Check sheet for the modelled part. Datum: model origin and axes. Units: mm. A direction names the side the tool comes from. Round coordinates to 2 decimals unless told otherwise and drop trailing zeros. Answer in a Markdown table with one row per item.
```python
from build123d import *

# Parameters (mm, degrees)
SKETCH_1_R          = 0.7
EXTRUDE_1_DEPTH     = 11
SKETCH_3_W          = 21.5
SKETCH_3_H          = 10
EXTRUDE_2_DEPTH     = 1.6
SKETCH_4_W          = 5
SKETCH_4_H          = 5
CUT_EXTRUDE_1_DEPTH = 1
CUT_EXTRUDE_2_REACH = 62.995
SKETCH_5_R          = 1.5
SKETCH_5_W          = 8
SKETCH_5_H          = 3
SKETCH_6_W          = 9.004768993
SKETCH_6_H          = 22
SKETCH_6_H_2        = 21.052305639
CUT_EXTRUDE_3_DEPTH = 1
SKETCH_7_W          = 5.5
SKETCH_7_H          = 20
SKETCH_7_W_2        = 4.9
SKETCH_7_W_3        = 2
SKETCH_7_H_2        = 2
EXTRUDE_4_DEPTH     = 2
FILLET_2_R          = 0.5
CUT_EXTRUDE_4_REACH = 62.994
SKETCH_9_R          = 5.5
FILLET_3_R          = 3


with BuildPart() as part:
    # Эскиз1 → Бобышка-Вытянуть1 (new body)
    with BuildSketch(Plane.XY):
        with BuildLine():
            Line((-15.979444254, 30.494289473), (15.979444254, 30.494289473))
            ThreePointArc((15.979444254, 30.494289473), (17.393657817, 29.908503035), (17.979444254, 28.494289473))
            Line((17.979444254, 28.494289473), (17.979444254, -28.500000343))
            ThreePointArc((17.979444254, -28.500000343), (17.393657817, -29.914213905), (15.979444254, -30.500000343))
            Line((15.979444254, -30.500000343), (-15.979444254, -30.500000343))
            ThreePointArc((-15.979444254, -30.500000343), (-17.393657817, -29.914213905), (-17.979444254, -28.500000343))
            Line((-17.979444254, -28.500000343), (-17.979444254, 28.494289473))
            ThreePointArc((-17.979444254, 28.494289473), (-17.393657817, 29.908503035), (-15.979444254, 30.494289473))
        make_face()
        with Locations((-15.979444254, 28.500000343)):
            Circle(SKETCH_1_R, mode=Mode.SUBTRACT)
        with Locations((16.01925313, 28.489204167)):
            Circle(SKETCH_1_R, mode=Mode.SUBTRACT)
        with Locations((16.028296267, -28.484120661)):
            Circle(SKETCH_1_R, mode=Mode.SUBTRACT)
        with Locations((-15.970396078, -28.505074873)):
            Circle(SKETCH_1_R, mode=Mode.SUBTRACT)
        with BuildLine():
            Line((-14.027975552, -29.00000033), (14.122849497, -29.00000033))
            ThreePointArc((14.122849497, -29.00000033), (14.623833191, -27.096913866), (16.520580958, -26.572442078))
            Line((16.520580958, -26.572442078), (16.520580958, 26.576499963))
            ThreePointArc((16.520580958, 26.576499963), (14.617623044, 27.094499874), (14.109055694, 29.00000033))
            Line((14.109055694, 29.00000033), (-14.044436107, 29.00000033))
            ThreePointArc((-14.044436107, 29.00000033), (-14.570671317, 27.074656136), (-16.499999911, 26.563221942))
            Line((-16.499999911, 26.563221942), (-16.499999911, -26.57182153))
            ThreePointArc((-16.499999911, -26.57182153), (-14.565751702, -27.075066872), (-14.027975552, -29.00000033))
        make_face(mode=Mode.SUBTRACT)
    extrude(amount=EXTRUDE_1_DEPTH)

    # Эскиз3 → Бобышка-Вытянуть2 (add)
    with BuildSketch(Plane.XY.offset(11)):
        with BuildLine():
            Line((-17.973934657, 28.494881466), (-17.973934657, -28.49940835))
            ThreePointArc((-17.973934657, -28.49940835), (-17.388148219, -29.913621912), (-15.973934657, -30.49940835))
            Line((-15.973934657, -30.49940835), (15.984953852, -30.49940835))
            ThreePointArc((15.984953852, -30.49940835), (17.399167415, -29.913621912), (17.984953852, -28.49940835))
            Line((17.984953852, -28.49940835), (17.984953852, 28.494881466))
            ThreePointArc((17.984953852, 28.494881466), (17.399167415, 29.909095028), (15.984953852, 30.494881466))
            Line((15.984953852, 30.494881466), (-15.973934657, 30.494881466))
            ThreePointArc((-15.973934657, 30.494881466), (-17.388148219, 29.909095028), (-17.973934657, 28.494881466))
        make_face()
        with Locations((0.015800122, -0.505118534)):
            Rectangle(SKETCH_3_W, SKETCH_3_H, mode=Mode.SUBTRACT)
    extrude(amount=-EXTRUDE_2_DEPTH)

    # Эскиз4 → Вырез-Вытянуть1 (cut)
    with BuildSketch(Plane.XY.offset(11)):
        with Locations((0.003657856, 9.994881549)):
            Rectangle(SKETCH_4_W, SKETCH_4_H)
    extrude(amount=-CUT_EXTRUDE_1_DEPTH, mode=Mode.SUBTRACT)

    # Эскиз5 → Вырез-Вытянуть2 (cut, up to next)
    with BuildSketch(Plane.XZ.offset(30.500000343), mode=Mode.PRIVATE) as cut_extrude_2_sk1:
        with Locations((-10.979444254, 2.5)):
            Circle(SKETCH_5_R)
    cut_extrude_2_tool1 = extrude(cut_extrude_2_sk1.sketch, amount=-CUT_EXTRUDE_2_REACH, mode=Mode.PRIVATE) & part.part
    add(cut_extrude_2_tool1.solids().sort_by_distance((-10.979444, -30.5, 2.5))[0], mode=Mode.SUBTRACT)
    # Эскиз5 → Вырез-Вытянуть2 (cut, up to next)
    with BuildSketch(Plane.XZ.offset(30.500000343), mode=Mode.PRIVATE) as cut_extrude_2_sk2:
        with Locations((7.979444254, 2.5)):
            Rectangle(SKETCH_5_W, SKETCH_5_H)
    cut_extrude_2_tool2 = extrude(cut_extrude_2_sk2.sketch, amount=-CUT_EXTRUDE_2_REACH, mode=Mode.PRIVATE) & part.part
    add(cut_extrude_2_tool2.solids().sort_by_distance((7.979444, -30.5, 2.5))[0], mode=Mode.SUBTRACT)

    # Эскиз6 → Вырез-Вытянуть3 (cut)
    with BuildSketch(Plane(origin=(0, 0, 9.4), x_dir=(-1, 0, 0), z_dir=(0, 0, -1))):
        with Locations((-0.015800121, 15.494881466)):
            Rectangle(SKETCH_6_W, SKETCH_6_H)
        with Locations((-0.015800121, -16.031271353)):
            Rectangle(SKETCH_6_W, SKETCH_6_H_2)
    extrude(amount=-CUT_EXTRUDE_3_DEPTH, mode=Mode.SUBTRACT)

    # Эскиз7 → Бобышка-Вытянуть4 (add)
    with BuildSketch(Plane(origin=(0, 0, 9.4), x_dir=(-1, 0, 0), z_dir=(0, 0, -1))):
        with Locations((-13.770580958, 3.3e-07)):
            Rectangle(SKETCH_7_W, SKETCH_7_H)
        with Locations((14.049999911, 3.3e-07)):
            Rectangle(SKETCH_7_W_2, SKETCH_7_H)
        with Locations((-5.520580958, 16.00000033)):
            Rectangle(SKETCH_7_W_3, SKETCH_7_H_2)
        Polygon((6.48268437, 17.014487668), (6.487140887, 15.014492633), (4.487145853, 15.010036116), (4.482689335, 17.01003115), align=None)
    extrude(amount=EXTRUDE_4_DEPTH)

    # Скругление2
    fillet_2_edges = [part.edges().sort_by_distance(p)[0] for p in [
        (16.520580958, 10.00000033, 8.4),
        (13.770580958, -9.99999967, 9.4),
        (16.520580958, -9.99999967, 8.4),
        (13.770580958, 10.00000033, 9.4),
        (16.520580958, 3.3e-07, 7.4),
        (11.020580958, 3.3e-07, 7.4),
        (-16.499999911, -9.99999967, 8.4),
        (-14.049999911, 10.00000033, 9.4),
        (-16.499999911, 10.00000033, 8.4),
        (-14.049999911, -9.99999967, 9.4),
        (-16.499999911, 3.3e-07, 7.4),
        (-11.599999911, 3.3e-07, 7.4),
        (6.520580958, 16.00000033, 9.4),
        (5.520580958, 17.00000033, 9.4),
        (5.520580958, 15.00000033, 7.4),
        (5.520580958, 17.00000033, 7.4),
        (-5.484634372, 17.012263749, 9.4),
        (-6.484912629, 16.014490151, 9.4),
        (-5.48714337, 15.012264374, 7.4),
    ]]
    fillet(fillet_2_edges, radius=FILLET_2_R)

    # Эскиз9 → Вырез-Вытянуть4 (cut, up to next)
    with BuildSketch(Plane(origin=(0, 30.494289473, 0), x_dir=(1, 0, 0), z_dir=(0, 1, 0)), mode=Mode.PRIVATE) as cut_extrude_4_sk1:
        with Locations((0, -3)):
            Circle(SKETCH_9_R)
    cut_extrude_4_tool1 = extrude(cut_extrude_4_sk1.sketch, amount=-CUT_EXTRUDE_4_REACH, mode=Mode.PRIVATE) & part.part
    add(cut_extrude_4_tool1.solids().sort_by_distance((0, 30.494289, 3))[0], mode=Mode.SUBTRACT)

    # Скругление3
    fillet_3_edges = [part.edges().sort_by_distance(p)[0] for p in [
        (4.609772229, 29.747144901, 0),
        (-4.609772229, 29.747144901, 0),
    ]]
    fillet(fillet_3_edges, radius=FILLET_3_R)


solid = part.part
```
(1) Tool access check on faces 1 (the flat face through (6.521, 16, 8)), 2 (the flat face through (8, -30, 1)), 3 (the flat face through (-0.1, -5.505, 10.6)), 4 (the flat face through (0, 30.494, 9)), 5 (the flat face through (3.979, -30, 2)). Record the directions out of +Z, -Z, +X, -X, +Y, -Y that give a thin tool (end or side, any length) a straight path to the whole face; none if there is none.
Solutions:
| item | result |
|---|---|
| face 1 | -Z |
| face 2 | -Y |
| face 3 | +Z, -Z |
| face 4 | +Z, -Z, +X, -X, +Y |
| face 5 | +Y, -Y |
(2) Depth check by flat-ended pin: pin 1 Ø0.8 at (x, y) = (-15.98, 28.5) entering from -Z; pin 2 Ø3.5 at (x, y) = (14, 2) entering from -Z; pin 3 Ø2.5 at (x, y) = (1.5, 14.5) entering from -Z. Enter the tip coordinate at first touch or a pass-through.
Solutions:
| item | result |
|---|---|
| pin 1 | z = 9.4 |
| pin 2 | z = 7.4 |
| pin 3 | z = 10.4 |
(3) Section check A-A on x = 0. Give the number of separate pieces and of enclosed holes in the cut face, plus the area to 3 significant figures.
Solutions:
| item | result |
|---|---|
| separate pieces | 3 |
| enclosed holes | 0 |
| area | 51.0 mm^2 |
(4) Scan lines: probe 1 along Y at (x, z) = (16, 3.5); probe 2 along X at (y, z) = (-14.5, 5.25); probe 3 along Y at (x, z) = (8.5, 9.5). Record each from-to range of solid material in increasing order. Write a range as from..to.
Solutions:
| item | result |
|---|---|
| probe 1 | -30.5..-29.18, -27.78..-26.51, 26.51..27.79, 29.19..30.49 |
| probe 2 | -17.98..-16.5, 16.52..17.98 |
| probe 3 | -30.5..-5.51, 4.49..30.49 |
(5) Draft check along Z on faces 6 (the flat face through (-5, 16, 7.4)), 7 (the flat face through (11.021, 0, 9)), 8 (the flat face through (8, -30, 4)). Enter one of: pulls with the +Z half, pulls with the -Z half, needs draft (parallel to the pull), parting line crosses it, or undercut.
Solutions:
| item | result |
|---|---|
| face 6 | pulls with the -Z half |
| face 7 | needs draft |
| face 8 | undercut |
